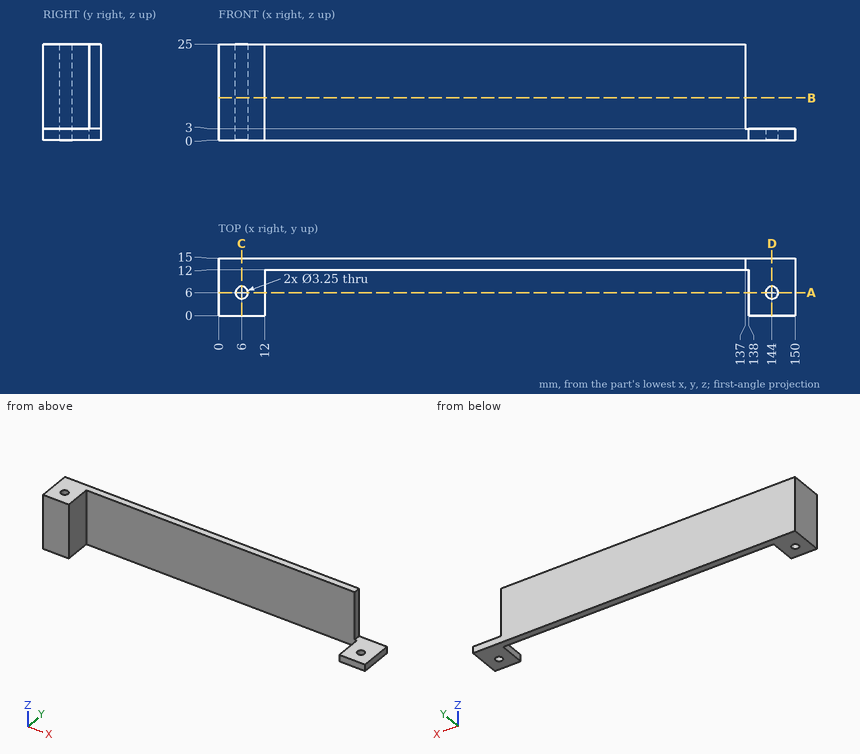
Source: three-view drawing plus pictorial views. Frame: mm from the lowest corner of the part. Round coordinates to 2 decimals unless told otherwise and drop trailing zeros. Write each loop counter-clockwise with the first axis right and the second up, starting at its lowest first coordinate (ties: lowest second). Pieces come first, ordered by that corner, then holes. Notation, with made-up numbers: M 41,7.5 L 71,7.5 A19 cw 71,18.5 Z; hole C 85.25,72 d6. An arc over 180 degrees is marked long. One line per item, written item: value. Start each with the question number.
Item 1: Section query C-C (x = 6). Return the cut outline in (y, z) (3 decimals).
Item 2: Section query B-B (z = 11). Return the cut outline in (x, y) (3 decimals), plus the area to 3 significant figures.
Item 3: Section query A-A (y = 6). Return the cut outline in (x, z) (3 decimals), plus the area to 3 significant figures.
Item 4: Ray query, L1, parallel to Y at x = 6, z = 8.75 (3 decimals); L2, parallel to X at y = 11.5, z = 12.5; L3, parallel to Y at x = 106.5, z = 4.75. Return the intervals inside material, ascending. Write a range as from..to.
Item 5: Pin query (flat end, axial travel): pin 1 (6.5 mm diameter, centred on x = 144.5, y = 5, fed in from +Z); pin 2 (1.5 mm diameter, centred on y = 13.5, z = 15.5, fed in from +X); pin 3 (2 mm diameter, centred on y = 4, z = 12, fed in from +X); pin 4 (3.5 mm diameter, centred on x = 144, y = 6, fed in from -Z). Return the tip coordinate at first contact, or that it passes through.
Item 6: Section query D-D (x = 144). Return the cut outline in (y, z) (3 decimals).
Result set:
1. outline: M 0,0 L 4.375,0 L 4.375,25 L 0,25 Z; M 7.625,0 L 15,0 L 15,25 L 7.625,25 Z
2. outline: M 0,0 L 12,0 L 12,12 L 137,12 L 137,15 L 0,15 Z; hole C 6,6 d3.25
2. area: 547 mm²
3. outline: M 0,0 L 4.375,0 L 4.375,25 L 0,25 Z; M 7.625,0 L 12,0 L 12,25 L 7.625,25 Z; M 138,0 L 142.375,0 L 142.375,3 L 138,3 Z; M 145.625,0 L 150,0 L 150,3 L 145.625,3 Z
3. area: 245 mm²
4. L1: y = 0..4.375, 7.625..15
4. L2: x = 0..12
4. L3: y = 12..15
5. pin 1: stops at z = 3
5. pin 2: stops at x = 137
5. pin 3: stops at x = 12
5. pin 4: stops at z = 0
6. outline: M 0,0 L 4.375,0 L 4.375,3 L 0,3 Z; M 7.625,0 L 15,0 L 15,3 L 7.625,3 Z
